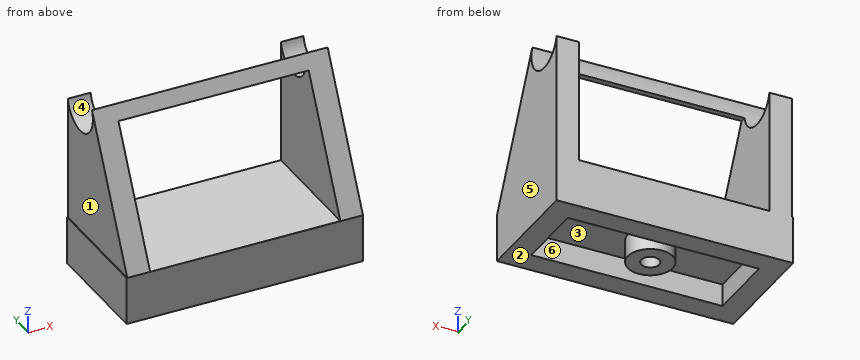
from build123d import *

# Parameters (mm, degrees)
F0_W      = 15.8
F0_H      = 7.8
F1_DEPTH  = 3.2
F3_DEPTH  = 1.5
F4_R      = 1.5020190756
F4_R_2    = 0.6083547137
F5_DEPTH  = 1.5
F7_DEPTH  = 15.75
F10_DEPTH = 25


# Not quite as in the source:
# - the program builds the solid bodies; features that only make, move or delete a surface that nothing else refers to are left out


with BuildPart() as f1:
    # F0 (on Top) → F1 (new body)
    with BuildSketch(Plane.XY):
        with Locations((-0.4272158258, 1.5226540988)):
            Rectangle(F0_W, F0_H)
    extrude(amount=F1_DEPTH)

    # F2 (on face) → F3 (cut)
    with BuildSketch(Plane(origin=(0, 0, 0), x_dir=(1, 0, 0), z_dir=(0, 0, -1))):
        Polygon((-0.8716915618, 0.8426669519), (-6.8171033636, 0.8426669519), (-6.8171033636, -1.5226540988), (-6.8171033636, -3.9279027842), (-0.4272158258, -3.9279027842), (5.9637515806, -3.9279027842), (5.9637515806, -1.5226540988), (5.9637515806, 0.8426669519), align=None)
    extrude(amount=-F3_DEPTH, mode=Mode.SUBTRACT)

    # F4 (on face) → F5 (join)
    with BuildSketch(Plane(origin=(0, 0, 1.5), x_dir=(1, 0, 0), z_dir=(0, 0, -1))):
        with Locations((-0.7097416674, -1.6585130943)):
            Circle(F4_R)
        with Locations((-0.7097416674, -1.6585130943)):
            Circle(F4_R_2, mode=Mode.SUBTRACT)
    extrude(amount=F5_DEPTH)

    # F6 (on face) → F7 (join)
    with BuildSketch(Plane.YZ.offset(7.4727841742)):
        with BuildLine():
            Line((-2.3773459012, 3.2), (5.4226540988, 3.2))
            Line((5.4226540988, 3.2), (5.4226540988, 11.4559076203))
            ThreePointArc((5.4226540988, 11.4559076203), (3.3247489231, 10.1865208896), (2.2503013028, 12.3906332074))
            Line((2.2503013028, 12.3906332074), (-2.3773459012, 3.2))
        make_face()
    extrude(amount=-F7_DEPTH)

    # F9 (on face) → F10 (cut)
    with BuildSketch(Plane(origin=(0, 5.4226540988, 0), x_dir=(-1, 0, 0), z_dir=(0, 1, 0))):
        Polygon((-5.9649683535, 11.4559076203), (-5.9649683535, 3.21011306), (6.7489589565, 3.2011167647), (6.7489589565, 11.4559076203), align=None)
    extrude(amount=-F10_DEPTH, mode=Mode.SUBTRACT)


solid = f1.part
The model under review builds one solid part; all positions refer to its coordinate system, in mm. Face numbers are marked on the shaded views. A direction names the side the tool comes from. Give positions to 0.01 mm unless a question says otherwise; leave off trailing zeros. Write each loop counter-clockwise with the first axis right and the second up, starting at its lowest first coordinate (ties: lowest second). Pieces come first, ordered by that corner, then holes.
1. Add section D-D, the plane y = 5.25. Write out the cut boundary in (x, z).
2. Add section A-A, the plane z = 4.25. Write out the cut boundary in (x, y).
3. For P1, Ø1.1, axis at x = -0.71, y = 1.66, coming from the +Z side; P2, Ø1, axis at x = 1, y = 0.5, coming from the -Z side, all flat-tipped, find the tip position at first contact; note any pin that passes through.
4. Draft analysis for pull direction X (two halves, no side actions). For the marked faces 4, 5 and 6, state which applies: +X half, -X half, draft (parallel to the pull), parting line (faces both ways), or undercut.
5. Add section C-C, the plane z = 6.25. Write out the cut boundary in (x, y), plus the area to 3 significant figures.
6. Wall thickness on L1, parallel to X at y = 1.5, z = 7; L2, parallel to Y at x = 1.5, z = 0.5; L3, parallel to Z at x = 3.25, y = -1.5: over which ranges is each line inside the solid? List them lowest first.
7. Tool access review of the marked faces 1, 2 and 3: name each direction out of +Z, -Z, +X, -X, +Y, -Y from which nothing blocks a thin tool from reaching the whole face with its end or side.
Worked answers:
1. outline: (-8.33, 0) - (7.47, 0) - (7.47, 10.98) - (5.96, 10.98) - (5.96, 3.21) - (-6.75, 3.2) - (-6.75, 10.98) - (-8.28, 10.98) - (-8.28, 3.2) - (-8.33, 3.2) - close
2. outline: (-8.28, -1.85) - (-6.75, -1.85) - (-6.75, 5.42) - (-8.28, 5.42) - close; (5.96, -1.85) - (7.47, -1.85) - (7.47, 5.42) - (5.96, 5.42) - close
3. P1: stops at z = 12.31
3. P2: stops at z = 1.5
4. face 4: draft
4. face 5: +X half
4. face 6: undercut
5. outline: (-8.28, -0.84) - (-6.75, -0.84) - (-6.75, 5.42) - (-8.28, 5.42) - close; (5.96, -0.84) - (7.47, -0.84) - (7.47, 5.42) - (5.96, 5.42) - close
5. area: 19.0 mm2
6. L1: x = -8.28 to -6.75, 5.96 to 7.47
6. L2: y = -2.38 to -0.84, 3.93 to 5.42
6. L3: z = 0 to 3.21
7. face 1: +Z, -X, +Y, -Y
7. face 2: -Z, +X, -X, +Y, -Y
7. face 3: -Z
